Can you work these out from the model? Positions are in its coordinate system, mm. Face numbers are marked on the shaded views. A direction names the side the tool comes from. Round coordinates to 2 decimals unless told otherwise and drop trailing zeros. Loops run counter-clockwise (first coordinate to the right, second up) from the corner with the lowest first, then second, coordinate; pieces in that order, holes last.
(1) Will these pins go through, and if not, where does the flat tip stop? pin 1 Ø4.5 at (x, y) = (-17.5, 13.5) entering from -Z; pin 2 Ø1 at (x, z) = (2.5, 1.5) entering from -Y; pin 3 Ø4 at (x, y) = (6, 11) entering from -Z.
(2) If I drill on line 1 along X through (y, z) = (11.75, 0); line 2 along Y through (x, z) = (-1, -0.7); line 3 along Z through (x, y) = (-0.5, 6.25), over which ranges is the centre line in solid material (lowest first)?
(3) I want a section at B-B on x = 3.5. Write out the boundary of the cut face in (y, z).
(4) I want a section at C-C on x = -9. Write out the boundary of the cut face in (y, z), plus the area to 3 significant figures.
(5) Thinking about a two-plate mould opening in X: for the marked faces 1, 2 and 3, which applies, released by +X, released by -X, zero draft, split by the parting line, or undercut?
(6) Which directions (+Z, -Z, +X, -X, +Y, -Y) give clear straight access to the entire face, cutting with the end or side of a thin tool? Please do the marked faces 4, 5, 6 and 7.
(7) I want a section at A-A on z = 1.05. Write out the boundary of the cut face in (x, y), plus the area to 3 significant figures.
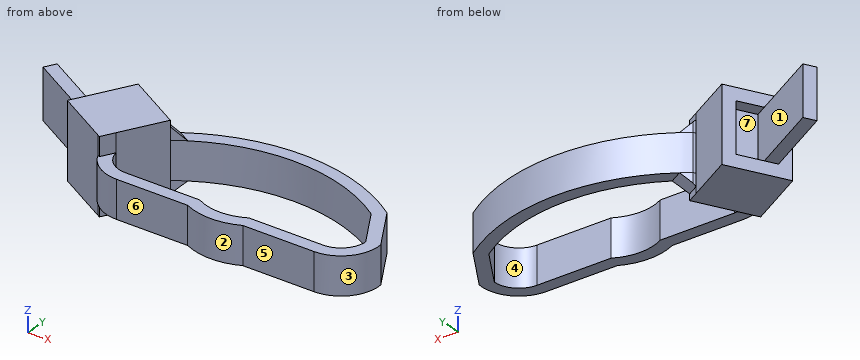
from build123d import *

# Parameters (mm, degrees)
BOSS_EXTRUDE2_DEPTH = 1.5
BOSS_EXTRUDE3_DEPTH = 3
SKETCH2_W           = 4
SKETCH2_H           = 1
BOSS_EXTRUDE4_DEPTH = 6
SKETCH2_3_W         = 4
SKETCH2_3_H         = 2
CUT_EXTRUDE1_DEPTH  = 1
CHAMFER1_SIZE       = 1


with BuildPart() as part:
    # Sketch1 → Boss-Extrude2 (new, symmetric)
    with BuildSketch(Plane.XY):
        with BuildLine():
            Line((-7.8, 6), (-2.179449472, 6))
            ThreePointArc((-2.179449472, 6), (0, 5.5), (2.179449472, 6))
            Line((2.179449472, 6), (7.8, 6))
            ThreePointArc((7.8, 6), (9.987434844, 6.946922115), (10.793982736, 9.189914132))
            Line((10.793982736, 9.189914132), (8.773900958, 12.688798406))
            ThreePointArc((8.773900958, 12.688798406), (0.077350269, 15.500303533), (-8.61920042, 12.688798406))
            Line((-8.61920042, 12.688798406), (-8.72820323, 12.5))
            Line((-8.72820323, 12.5), (-7.862177826, 12))
            ThreePointArc((-7.862177826, 12), (0.077350269, 14.500303533), (8.016878365, 12))
            Line((8.016878365, 12), (9.798179943, 8.914695163))
            ThreePointArc((9.798179943, 8.914695163), (9.183725104, 7.55594154), (7.8, 7))
            Line((7.8, 7), (1.936491673, 7))
            ThreePointArc((1.936491673, 7), (0, 6.5), (-1.936491673, 7))
            Line((-1.936491673, 7), (-7.8, 7))
            ThreePointArc((-7.8, 7), (-9.098627684, 7.478958864), (-9.775266128, 8.686433862))
            Line((-9.775266128, 8.686433862), (-10.362177826, 7.669872981))
            Line((-10.362177826, 7.669872981), (-10.536485592, 7.770509617))
            ThreePointArc((-10.536485592, 7.770509617), (-9.429651627, 6.481223397), (-7.8, 6))
        make_face()
    extrude(amount=BOSS_EXTRUDE2_DEPTH, both=True)

    # Sketch1<5> → Boss-Extrude3 (add, symmetric)
    with BuildSketch(Plane.XY):
        with BuildLine():
            Line((-14.692304845, 10.169872981), (-10.536485592, 7.770509617))
            ThreePointArc((-10.536485592, 7.770509617), (-10.724033666, 8.329159391), (-10.798758273, 8.913693465))
            Line((-10.798758273, 8.913693465), (-8.72820323, 12.5))
            Line((-8.72820323, 12.5), (-12.192304845, 14.5))
            Line((-12.192304845, 14.5), (-14.692304845, 10.169872981))
        make_face()
        with BuildLine():
            ThreePointArc((-10.798758273, 8.913693465), (-10.724033666, 8.329159391), (-10.536485592, 7.770509617))
            Line((-10.536485592, 7.770509617), (-10.362177826, 7.669872981))
            Line((-10.362177826, 7.669872981), (-9.775266128, 8.686433862))
            Line((-9.775266128, 8.686433862), (-7.862177826, 12))
            Line((-7.862177826, 12), (-8.72820323, 12.5))
            Line((-8.72820323, 12.5), (-10.798758273, 8.913693465))
        make_face()
    extrude(amount=BOSS_EXTRUDE3_DEPTH, both=True)

    # Sketch2 → Boss-Extrude4 (add)
    with BuildSketch(Plane(origin=(-15.422912811, 8.904422863, 0), x_dir=(0, 0, 1), z_dir=(-0.8660254037844408, 0.4999999999999963, 0))):
        with Locations((0, 2.961215932)):
            Rectangle(SKETCH2_W, SKETCH2_H)
    extrude(amount=BOSS_EXTRUDE4_DEPTH)

    # Sketch2<3> → Cut-Extrude1 (cut)
    with BuildSketch(Plane(origin=(-15.422912811, 8.904422863, 0), x_dir=(0, 0, 1), z_dir=(-0.8660254037844408, 0.4999999999999963, 0))):
        with Locations((0, 4.461215932)):
            Rectangle(SKETCH2_3_W, SKETCH2_3_H)
    extrude(amount=-CUT_EXTRUDE1_DEPTH, mode=Mode.SUBTRACT)

    # Chamfer1
    # the kernel refuses this chamfer: 1 mm, written as the material it adds along each edge
    with BuildSketch(Plane(origin=(-8.72820323, 12.5, -1.5), x_dir=(0.4998109584556448, 0.8656979742248824, 0.027495876610586233), z_dir=(0.8660254037844407, -0.4999999999999965, 0))) as chamfer1_piece_1_section:
        Polygon((CHAMFER1_SIZE * 0.999621916911, -CHAMFER1_SIZE * 0.0274958766106), (-CHAMFER1_SIZE * 0.0274958766106, -CHAMFER1_SIZE * 0.999621916911), (0, 0), align=None)
    chamfer1_piece_1 = extrude(amount=1, mode=Mode.PRIVATE)
    chamfer1_piece_1 = chamfer1_piece_1 & Plane(origin=(0.077350269, 0.64446099, -1.842899674), x_dir=(0.5853959924126673, 0.8107475143762012, 0), z_dir=(0, 0, 1)) * Cylinder(14.855842544, 6, mode=Mode.PRIVATE)
    chamfer1_piece_1 = chamfer1_piece_1 - Plane(origin=(0.077350269, 0.64446099, -1.842899674), x_dir=(-0.5730094052913434, 0.8195487913770974, 0), z_dir=(0, 0, 1)) * Cylinder(13.855842544, 6, mode=Mode.PRIVATE)
    add(chamfer1_piece_1)
    with BuildSketch(Plane(origin=(-8.72820323, 12.5, -1.5), x_dir=(0.4998109584556448, 0.8656979742248824, 0.027495876610586233), z_dir=(0.8660254037844407, -0.4999999999999965, 0))) as chamfer1_piece_2_section:
        Polygon((CHAMFER1_SIZE * 0.999621916911, -CHAMFER1_SIZE * 0.0274958766106), (-CHAMFER1_SIZE * 0.0274958766106, -CHAMFER1_SIZE * 0.999621916911), (0, 0), align=None)
    chamfer1_piece_2 = extrude(amount=3.571682988, mode=Mode.PRIVATE)
    chamfer1_piece_2 = split(chamfer1_piece_2, bisect_by=Plane(origin=(-7.598721959, 12.456318948, -1.72489745), z_dir=(0.8660254037844384, -0.5000000000000004, 0)), keep=Keep.TOP, mode=Mode.PRIVATE)
    chamfer1_piece_2 = chamfer1_piece_2 - Plane(origin=(0.077350269, 0.64446099, -1.72489745), x_dir=(-0.5730094052913434, 0.8195487913770974, 0), z_dir=(0, 0, 1)) * Cylinder(13.855842544, 12, mode=Mode.PRIVATE)
    add(chamfer1_piece_2)
    with BuildSketch(Plane(origin=(-8.72820323, 12.5, 1.5), x_dir=(0.4998109584556448, 0.8656979742248824, -0.027495876610586233), z_dir=(0.8660254037844407, -0.4999999999999965, 0))) as chamfer1_piece_3_section:
        Polygon((CHAMFER1_SIZE * 0.999621916911, CHAMFER1_SIZE * 0.0274958766106), (-CHAMFER1_SIZE * 0.0274958766106, CHAMFER1_SIZE * 0.999621916911), (0, 0), align=None)
    chamfer1_piece_3 = extrude(amount=1, mode=Mode.PRIVATE)
    chamfer1_piece_3 = chamfer1_piece_3 & Plane(origin=(0.077350269, 0.64446099, 1.842899674), x_dir=(0.5853959924126673, 0.8107475143762012, 0), z_dir=(0, 0, 1)) * Cylinder(14.855842544, 6, mode=Mode.PRIVATE)
    chamfer1_piece_3 = chamfer1_piece_3 - Plane(origin=(0.077350269, 0.64446099, 1.842899674), x_dir=(-0.5730094052913434, 0.8195487913770974, 0), z_dir=(0, 0, 1)) * Cylinder(13.855842544, 6, mode=Mode.PRIVATE)
    add(chamfer1_piece_3)
    with BuildSketch(Plane(origin=(-8.72820323, 12.5, 1.5), x_dir=(0.4998109584556448, 0.8656979742248824, -0.027495876610586233), z_dir=(0.8660254037844407, -0.4999999999999965, 0))) as chamfer1_piece_4_section:
        Polygon((CHAMFER1_SIZE * 0.999621916911, CHAMFER1_SIZE * 0.0274958766106), (-CHAMFER1_SIZE * 0.0274958766106, CHAMFER1_SIZE * 0.999621916911), (0, 0), align=None)
    chamfer1_piece_4 = extrude(amount=3.571682988, mode=Mode.PRIVATE)
    chamfer1_piece_4 = split(chamfer1_piece_4, bisect_by=Plane(origin=(-7.598721959, 12.456318948, 1.72489745), z_dir=(0.8660254037844384, -0.5000000000000004, 0)), keep=Keep.TOP, mode=Mode.PRIVATE)
    chamfer1_piece_4 = chamfer1_piece_4 - Plane(origin=(0.077350269, 0.64446099, 1.72489745), x_dir=(-0.5730094052913434, 0.8195487913770974, 0), z_dir=(0, 0, 1)) * Cylinder(13.855842544, 12, mode=Mode.PRIVATE)
    add(chamfer1_piece_4)


solid = part.part
Filled sheet:
1. pin 1: stops at z = -2
1. pin 2: stops at y = 5.92
1. pin 3: stops at z = -1.5
2. line 1: x = -15.43 to -13.43, -12.63 to -8.01, 8.16 to 9.32
2. line 2: y = 5.6 to 6.63, 14.46 to 15.46
2. line 3: z = -1.5 to 1.5
3. outline: (6, -1.5) - (7, -1.5) - (7, 1.5) - (6, 1.5) - close; (14.07, -1.5) - (15.1, -1.5) - (15.1, 1.5) - (14.07, 1.5) - close
4. outline: (6.25, -1.5) - (7.4, -1.5) - (7.4, 1.5) - (6.25, 1.5) - close; (10.03, -3) - (12.66, -3) - (12.66, 3) - (10.03, 3) - close
4. area: 19.2 mm2
5. face 1: undercut
5. face 2: split by the parting line
5. face 3: released by +X
6. face 4: +Z, -Z
6. face 5: +Z, -Z, +X, -Y
6. face 6: +Z, -Z, -X, -Y
6. face 7: none
7. outline: (-19.39, 14.04) - (-14.19, 11.04) - (-14.69, 10.17) - (-10.54, 7.77) arc R3 ccw to (-7.8, 6) - (-2.18, 6) arc R5 ccw to (2.18, 6) - (7.8, 6) arc R3 ccw to (10.79, 9.19) - (8.77, 12.69) arc R14.86 ccw to (-8.62, 12.69) - (-8.73, 12.5) - (-12.19, 14.5) - (-12.69, 13.63) - (-11.83, 13.13) - (-12.83, 11.4) - (-18.89, 14.9) - close; hole (-9.78, 8.69) arc R2 ccw to (-7.8, 7) - (-1.94, 7) arc R4 ccw to (1.94, 7) - (7.8, 7) arc R2 ccw to (9.8, 8.91) - (8.02, 12) arc R13.86 ccw to (-7.86, 12) - close
7. area: 73.4 mm2
